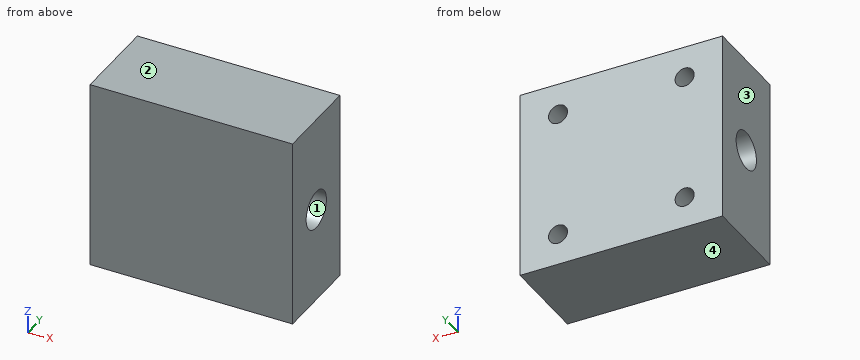
```python
from build123d import *

# Parameters (mm, degrees)
SKETCH_1_W          = 32
SKETCH_1_H          = 14
EXTRUDE_1_DEPTH     = 30
SKETCH_2_R          = 1.5
CUT_EXTRUDE_1_DEPTH = 10
CUT_EXTRUDE_2_REACH = 46.418
SKETCH_3_R          = 3


with BuildPart() as part:
    # 草图1 → 凸台-拉伸1 (new body)
    with BuildSketch(Plane.XY):
        Rectangle(SKETCH_1_W, SKETCH_1_H)
    extrude(amount=-EXTRUDE_1_DEPTH)

    # 草图2 → 切除-拉伸1 (cut)
    with BuildSketch(Plane(origin=(0, 7, 0), x_dir=(1, 0, 0), z_dir=(0, 1, 0))):
        with Locations(Location((-10, 25, 0), (0, 0, 270))):
            Circle(SKETCH_2_R)
        with Locations(Location((10, 25, 0), (0, 0, 90))):
            Circle(SKETCH_2_R)
        with Locations(Location((10, 5, 0), (0, 0, 270))):
            Circle(SKETCH_2_R)
        with Locations(Location((-10, 5, 0), (0, 0, 90))):
            Circle(SKETCH_2_R)
    extrude(amount=-CUT_EXTRUDE_1_DEPTH, mode=Mode.SUBTRACT)

    # 草图3 → 切除-拉伸2 (cut, up to next)
    with BuildSketch(Plane(origin=(16, 0, 0), x_dir=(0, 0, -1), z_dir=(1, 0, 0)), mode=Mode.PRIVATE) as cut_extrude_2_sk1:
        with Locations((15, 0)):
            Circle(SKETCH_3_R)
    cut_extrude_2_tool1 = extrude(cut_extrude_2_sk1.sketch, amount=-CUT_EXTRUDE_2_REACH, mode=Mode.PRIVATE) & part.part
    add(cut_extrude_2_tool1.solids().sort_by_distance((16, 0, -15))[0], mode=Mode.SUBTRACT)


solid = part.part
```
CAD build for the part. Positions are in the model's coordinates, mm. Face numbers are marked on the shaded views. Coordinates: 2 decimals unless noted, no trailing zeros. Loops run counter-clockwise (first coordinate to the right, second up) from the corner with the lowest first, then second, coordinate; pieces in that order, holes last. Notation, with made-up numbers: (-28, 76) - (-21, 76) arc R33 cw to (-21, 104) - close; hole circle Ø11 at (-3.5, 26.5). An arc over 180 degrees is marked (long way). Use CSV: the item, a comma, the result in double quotes. Start each with the question number.
Q1. Two-plate mould, pull along Z, no slides. Class the marked faces 1, 2, 3 and 4: +Z half, -Z half, draft (parallel to the pull), parting line (faces both ways), or undercut.
Q2. Probe probe 1 along X at (y, z) = (-0.5, -5); probe 2 along Y at (x, z) = (10, -15); probe 3 along Z at (x, y) = (9, 4.5). List the from-to ranges inside material, lowest first. Write a range as from..to.
Q3. Cut at B-B, the plane z = -15. List the corners of the cut face in (x, y).
Q4. Cut at D-D, the plane y = 5.75. List the corners of the cut face in (x, z), then the cut area to 3 significant figures.
Q5. Drop flat-ended pins along their axis: P1, Ø1.5, axis at x = -10.5, z = -24.5, coming from the +Y side; P2, Ø8, axis at y = 0, z = -15, coming from the -X side. Give the stop position or say it passes through.
Q6. Cut at A-A, the plane y = 0. List the corners of the cut face in (x, z).
Q7. Cut at C-C, the plane x = -10. List the corners of the cut face in (y, z).
Here are the results:
1,face 1,"undercut"
1,face 2,"+Z half"
1,face 3,"draft"
1,face 4,"-Z half"
2,probe 1,"-16..-11.5, -8.5..8.5, 11.5..16"
2,probe 2,"-7..-3, 3..7"
2,probe 3,"-30..-26.12, -23.88..-6.12, -3.88..0"
3,outline,"(-16, -7) - (16, -7) - (16, -3) - (-16, -3) - close; (-16, 3) - (16, 3) - (16, 7) - (-16, 7) - close"
4,outline,"(-16, -30) - (16, -30) - (16, 0) - (-16, 0) - close; hole circle Ø3 at (-10, -25); hole circle Ø3 at (-10, -5); hole circle Ø3 at (10, -25); hole circle Ø3 at (10, -5)"
4,area,"932 mm2"
5,P1,"y = -3"
5,P2,"x = -16"
6,outline,"(-16, -30) - (16, -30) - (16, -18) - (-16, -18) - close; (-16, -12) - (16, -12) - (16, 0) - (-16, 0) - close; hole circle Ø3 at (-10, -25); hole circle Ø3 at (-10, -5); hole circle Ø3 at (10, -25); hole circle Ø3 at (10, -5)"
7,outline,"(-7, -30) - (7, -30) - (7, -26.5) - (-3, -26.5) - (-3, -23.5) - (7, -23.5) - (7, -6.5) - (-3, -6.5) - (-3, -3.5) - (7, -3.5) - (7, 0) - (-7, 0) - close; hole circle Ø6 at (0, -15)"
